Read the model definition and answer for the solid it produces. Units are mm, in the model's axes. Round coordinates to 2 decimals unless told otherwise and drop trailing zeros. Order: outer loops, then holes, each group sorted by start corner. A loop starts at its lowest first (then second) coordinate and runs counter-clockwise, first axis right, second up. Notation, with made-up numbers: (37, 24) - (45, 24) arc R27 cw to (45, 43) - close; hole circle Ø4 at (23.25, 57.25). An arc over 180 degrees is marked (long way). One line per question, with ' | ' between items. Start each with the question number.
1) The part is cut by section A-A, the plane x = -3. Give the vertices of the cut face in (y, z).
2) The mould has two halves that part along Y. Classify faces 1 (the flat face through (-29.577, 19.72, 22.185)), 2 (the cylindrical face through (-4.97, 20.29, 22.19)), 3 (the flat face through (-13.366, 37.598, 22.185)): pulls with the +Y half, pulls with the -Y half, needs draft (parallel to the pull), parting line crosses it, or undercut.
3) Flat-ended cylindrical pins translate along their axes: pin 1 (5 mm diameter, centred on x = -6, z = 17.5, fed in from -Y); pin 2 (10 mm diameter, centred on y = 15.5, z = 19.5, fed in from +X); pin 3 (6 mm diameter, centred on y = 20, z = 13, fed in from +X). Find the tip coordinate at first contact, or state that the pin passes through.
4) Straight lines are drawn through the part: line 1 (X direction, y = 25, z = 18); line 2 (X direction, y = 18.5, z = 20.5); line 3 (Y direction, x = -8.5, z = 3). For each, find the intervals that lie inside material, in ascending order. Write a range as from..to.
5) The part is cut by section B-B, the plane y = 20.5. Give the vertices of the cut face in (x, z), plus the area to 3 significant figures.
6) The part is cut by section C-C, the plane z = 21. Give the vertices of the cut face in (x, y), plus the area to 3 significant figures.
from build123d import *

# Parameters (mm, degrees)
F1_DEPTH = 35
F3_DEPTH = 40.001
F5_DEPTH = 45.001


with BuildPart() as f1:
    # F0 (on Right) → F1 (new body)
    with BuildSketch(Plane.YZ):
        Polygon((5.127102, 45), (0, 0), (40, 0), (35.127102, 45), align=None)
    extrude(amount=-F1_DEPTH)

    # F2 (on Front) → F3 (cut, through all)
    with BuildSketch(Plane.XZ):
        Polygon((-35, 45), (-35, 0), (-24, 45), align=None)
    extrude(amount=-F3_DEPTH, mode=Mode.SUBTRACT)

    # F4 (on Top) → F5 (cut, through all)
    with BuildSketch(Plane.XY):
        with BuildLine():
            Line((0, 0), (0, 40))
            ThreePointArc((0, 40), (-4.972394, 20), (0, 0))
        make_face()
    extrude(amount=F5_DEPTH, mode=Mode.SUBTRACT)


solid = f1.part
Values:
1) outline: (0, 0) - (7.17, 0) - (7.17, 45) - (5.13, 45) - close; (32.83, 0) - (40, 0) - (35.13, 45) - (32.83, 45) - close
2) face 1: needs draft | face 2: undercut | face 3: pulls with the +Y half
3) pin 1: stops at y = 1.71 | pin 2: stops at x = -3.9 | pin 3: stops at x = -4.87
4) line 1: x = -30.6..-4.68 | line 2: x = -29.99..-4.95 | line 3: y = 0.34..39.68
5) outline: (-35, 0) - (-4.97, 0) - (-4.97, 45) - (-24, 45) - close | area: 1,100 mm^2
6) outline: (-29.87, 2.39) - (-1.17, 2.39) arc R42.71 cw to (-1.12, 37.73) - (-29.87, 37.73) - close | area: 924 mm^2
